CAD build for the part. Positions are in the model's coordinates, mm. Face numbers are marked on the shaded views. A direction names the side the tool comes from. Round coordinates to 2 decimals unless told otherwise and drop trailing zeros. Order: outer loops, then holes, each group sorted by start corner. A loop starts at its lowest first (then second) coordinate and runs counter-clockwise, first axis right, second up. Notation, with made-up numbers: M 33,-23 L 43,-23 A28 cw 43,0 Z; hole C -3.5,62.25 d3. An arc over 180 degrees is marked long. Answer as a JSON object with one key per item and string values. Group by question number.
```python
from build123d import *

# Parameters (mm, degrees)
F0_W     = 203.2
F0_H     = 101.6
F1_DEPTH = 101.6
F2_W     = 76.2
F2_H     = 101.6
F3_DEPTH = 50.8
F6_DEPTH = 25.4


with BuildPart() as f1:
    # F0 (on Top) → F1 (new body)
    with BuildSketch(Plane.XY):
        with Locations((-39.355746, 19.929246)):
            Rectangle(F0_W, F0_H)
    extrude(amount=F1_DEPTH)

    # F2 (on face) → F3 (cut)
    with BuildSketch(Plane.XY.offset(101.6)):
        with Locations((24.144254, 19.929246)):
            Rectangle(F2_W, F2_H)
    extrude(amount=-F3_DEPTH, mode=Mode.SUBTRACT)

    # F5 (on face) → F6 (cut)
    with BuildSketch(Plane.XY.offset(101.6)):
        Polygon((-140.955746, 70.729246), (-140.955746, 70.360331), (-15.061975, 70.360331), (-15.061975, 44.960331), (-140.955746, 44.960331), (-140.955746, -5.470754), (-13.955746, -5.470754), (-13.955746, 70.729246), align=None)
    extrude(amount=-F6_DEPTH, mode=Mode.SUBTRACT)


solid = f1.part
```
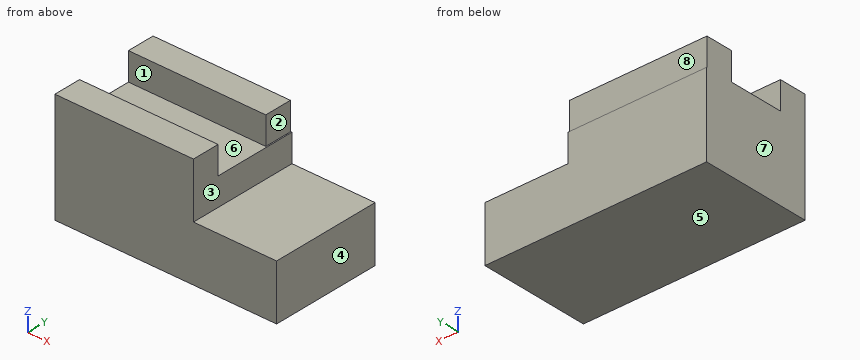
Item 1: 3-axis set-ups, long thin cutter, end or side, ignore diameter. For the marked faces 1, 2, 3, 4 and 5: which of +Z, -Z, +X, -X, +Y, -Y reach the whole face in a straight line?
Item 2: Cut at C-C, the plane y = -1.5. Give the cut face in (x, z), and give its area (3 significant figures).
Item 3: Cut at B-B, the plane x = -62.5. Give the cut face in (y, z), and give its area (3 significant figures).
Item 4: Drill centre lines: line 1 (X direction, y = 26.5, z = 71.5); line 2 (Y direction, x = -117.5, z = 91.5); line 3 (Z direction, x = -8.5, y = 57.5). Where is each one in solid material? Low to high. Write a range as [from, to].
Item 5: Two-plate mould, pull along Y, no slides. Class the marked faces 6, 7 and 8: +Y half, -Y half, draft (parallel to the pull), parting line (faces both ways), or undercut.
Item 6: Cut at D-D, the plane y = -18. Give the cut face in (x, z).
Item 7: Flat gauge pins, fed straight in: pin 1 Ø7.5 at (x, z) = (-56, 92) entering from +Y; pin 2 Ø20.5 at (y, z) = (63.5, 86.5) entering from +X; pin 3 Ø15 at (y, z) = (-5.5, 72) entering from +X. Where does each tip first touch, or does it go through?
Item 8: Cut at A-A, the plane z = 86. Give the cut face in (x, y), and give its area (3 significant figures).
Response values:
{
 "1": {"face 1": "+Z, +X, -X", "face 2": "+Z, +X, +Y", "face 3": "+Z, +X, +Y, -Y", "face 4": "+Z, -Z, +X, +Y, -Y", "face 5": "-Z, +X, -X, +Y, -Y"},
 "2": {"outline": "M -140.96,0 L 62.24,0 L 62.24,50.8 L -13.96,50.8 L -13.96,76.2 L -140.96,76.2 Z", "area": "13,500 mm^2"},
 "3": {"outline": "M -30.87,0 L 70.73,0 L 70.73,76.2 L 70.36,76.2 L 70.36,101.6 L 44.96,101.6 L 44.96,76.2 L -5.47,76.2 L -5.47,101.6 L -30.87,101.6 Z", "area": "9,030 mm^2"},
 "4": {"line 1": "[-140.96, -13.96]", "line 2": "[-30.87, -5.47], [44.96, 70.36]", "line 3": "[0, 50.8]"},
 "5": {"face 6": "undercut", "face 7": "draft", "face 8": "+Y half"},
 "6": {"outline": "M -140.96,0 L 62.24,0 L 62.24,50.8 L -13.96,50.8 L -13.96,101.6 L -140.96,101.6 Z"},
 "7": {"pin 1": "y = 70.36", "pin 2": "x = -15.06", "pin 3": "x = -13.96"},
 "8": {"outline": "M -140.96,-30.87 L -13.96,-30.87 L -13.96,-5.47 L -140.96,-5.47 Z; M -140.96,44.96 L -15.06,44.96 L -15.06,70.36 L -140.96,70.36 Z", "area": "6,420 mm^2"}
}
